Input: part model. Units: mm. Frame: model coordinates. Give positions to 0.01 mm unless a question says otherwise; leave off trailing zeros. Order: outer loops, then holes, each group sorted by start corner. A loop starts at its lowest first (then second) coordinate and runs counter-clockwise, first axis right, second up. Notation, with made-up numbers: M 56.25,4 L 64.25,4 A13 ccw 64.25,23 Z; hole C 59.5,-25 d2. An arc over 180 degrees is marked long. Use a Markdown table: item, result.
from build123d import *

# Parameters (mm, degrees)
SKETCH1_R           = 25
BOSS_EXTRUDE1_DEPTH = 10
CHAMFER1_SIZE       = 2


with BuildPart() as part:
    # Sketch1 → Boss-Extrude1 (new, symmetric)
    with BuildSketch(Plane.YZ):
        with BuildLine():
            Line((94.677868983, -37.128576072), (-94.677868983, -37.128576072))
            ThreePointArc((-94.677868983, -37.128576072), (-131.806445055, 0), (-94.677868983, 37.128576072))
            Line((-94.677868983, 37.128576072), (94.677868983, 37.128576072))
            ThreePointArc((94.677868983, 37.128576072), (131.806445055, 0), (94.677868983, -37.128576072))
        make_face()
        with Locations(Location((-94.677868983, 0, 0), (0, 0, 270))):
            Circle(SKETCH1_R, mode=Mode.SUBTRACT)
        with Locations(Location((94.677868983, 0, 0), (0, 0, 270))):
            Circle(SKETCH1_R, mode=Mode.SUBTRACT)
    extrude(amount=BOSS_EXTRUDE1_DEPTH, both=True)

    # Chamfer1
    chamfer1_edges = [part.edges().sort_by_distance(p)[0] for p in [
        (10, -131.806445055, 0),
        (10, 0, -37.128576072),
        (10, 131.806445055, 0),
        (-10, 0, -37.128576072),
        (-10, -131.806445055, 0),
        (-10, 0, 37.128576072),
        (-10, 131.806445055, 0),
        (10, 0, 37.128576072),
    ]]
    chamfer(chamfer1_edges, length=CHAMFER1_SIZE)


solid = part.part
1) Cut plane A-A on z = 0. Return loops of the section in (x, y), and give its area (3 significant figures).
Response values:
| item | result |
|---|---|
| outline | M -10,-129.81 L -8,-131.81 L 8,-131.81 L 10,-129.81 L 10,-119.68 L -10,-119.68 Z; M -10,-69.68 L 10,-69.68 L 10,69.68 L -10,69.68 Z; M -10,119.68 L 10,119.68 L 10,129.81 L 8,131.81 L -8,131.81 L -10,129.81 Z |
| area | 3,260 mm² |
2) Material intervals for line 1 (Y direction, x = 5.5, z = 0); line 2 (Y direction, x = 0, z = -1.5); line 3 (Z direction, x = 1, y = -94), sorted ascending. Write a range as from..to.
Response values:
| item | result |
|---|---|
| line 1 | y = -131.81..-119.68, -69.68..69.68, 119.68..131.81 |
| line 2 | y = -131.78..-119.63, -69.72..69.72, 119.63..131.78 |
| line 3 | z = -37.13..-24.99, 24.99..37.13 |
3) Cut plane C-C on y = -88. Return loops of the section in (x, z).
Response values:
| item | result |
|---|---|
| outline | M -10,-35.13 L -8,-37.13 L 8,-37.13 L 10,-35.13 L 10,-24.09 L -10,-24.09 Z; M -10,24.09 L 10,24.09 L 10,35.13 L 8,37.13 L -8,37.13 L -10,35.13 Z |
4) Cut plane D-D on y = 76. Return loops of the section in (x, z).
Response values:
| item | result |
|---|---|
| outline | M -10,-35.13 L -8,-37.13 L 8,-37.13 L 10,-35.13 L 10,-16.62 L -10,-16.62 Z; M -10,16.62 L 10,16.62 L 10,35.13 L 8,37.13 L -8,37.13 L -10,35.13 Z |
5) Cut plane B-B on x = -3.5. Return loops of the section in (y, z), and give its area (3 significant figures).
Response values:
| item | result |
|---|---|
| outline | M -94.68,-37.13 L 94.68,-37.13 A37.13 ccw 94.68,37.13 L -94.68,37.13 A37.13 ccw Z; hole C -94.68,0 d50; hole C 94.68,0 d50 |
| area | 14,500 mm² |
6) Mould query, pull axis Z, two halves, no side actions, for faces 1 (the face through (-9.7, -130.1, -0.8)), 2 (the face through (-10, 2, 0)), 3 (the face through (-0.14, -87.169, -23.846)). Classes: released by +Z, released by -Z, zero draft, split by the parting line, or undercut.
Response values:
| item | result |
|---|---|
| face 1 | split by the parting line |
| face 2 | zero draft |
| face 3 | undercut |
7) First-contact query: pin 1 Ø4 at (x, z) = (-5, 8.5) entering from +Y. Flat tip, straight axial feed; report the tip coordinate or a pass-through.
Response values:
| item | result |
|---|---|
| pin 1 | stops at y = 131.23 |
